Job drawing, mm, ordinate dimensions from the low corner. One solid piece. A direction names the side the tool comes from. Give positions to 0.01 mm unless a question says otherwise; leave off trailing zeros. Order: outer loops, then holes, each group sorted by start corner. A loop starts at its lowest first (then second) coordinate and runs counter-clockwise, first axis right, second up. Notation, with made-up numbers: M 27,-38 L 41,-38 A7 cw 41,-25 Z; hole C -4,43 d5. An arc over 180 degrees is marked long. Put each result on its own line as item: value. Start each with the question number.
1) Cut at D-D (z = 7.25). Write the cut outline in (x, y) (3 decimals), and give its area (3 significant figures).
2) Tool access for the marked faces 1 and 2: list every direction of +Z, -Z, +X, -X, +Y, -Y with a clear straight run to the whole face (end or side of a thin tool).
3) Two-plate mould, pull along Y, no slides. Class the marked faces 3, 4, 5 and 6: released by +Y, released by -Y, zero draft, split by the parting line, or undercut.
4) Pin check, flat tips, straight feed: pin 1 (3 mm diameter, centred on x = 4, z = 6.5, fed in from -Y); pin 2 (3 mm diameter, centred on x = 16.5, z = 5, fed in from -Y); pin 3 (2 mm diameter, centred on y = 6, z = 5.5, fed in from -X). Stop position of each tip, or through.
5) Cut at C-C (z = 4.25). Write the cut outline in (x, y).
6) Drill centre lines: line 1 (Z direction, x = 7.5, y = 11); line 2 (Z direction, x = 13.75, y = 3.5); line 3 (X direction, y = 8.25, z = 2.25). Where is each one in solid material? Low to high. Write a range as [from, to].
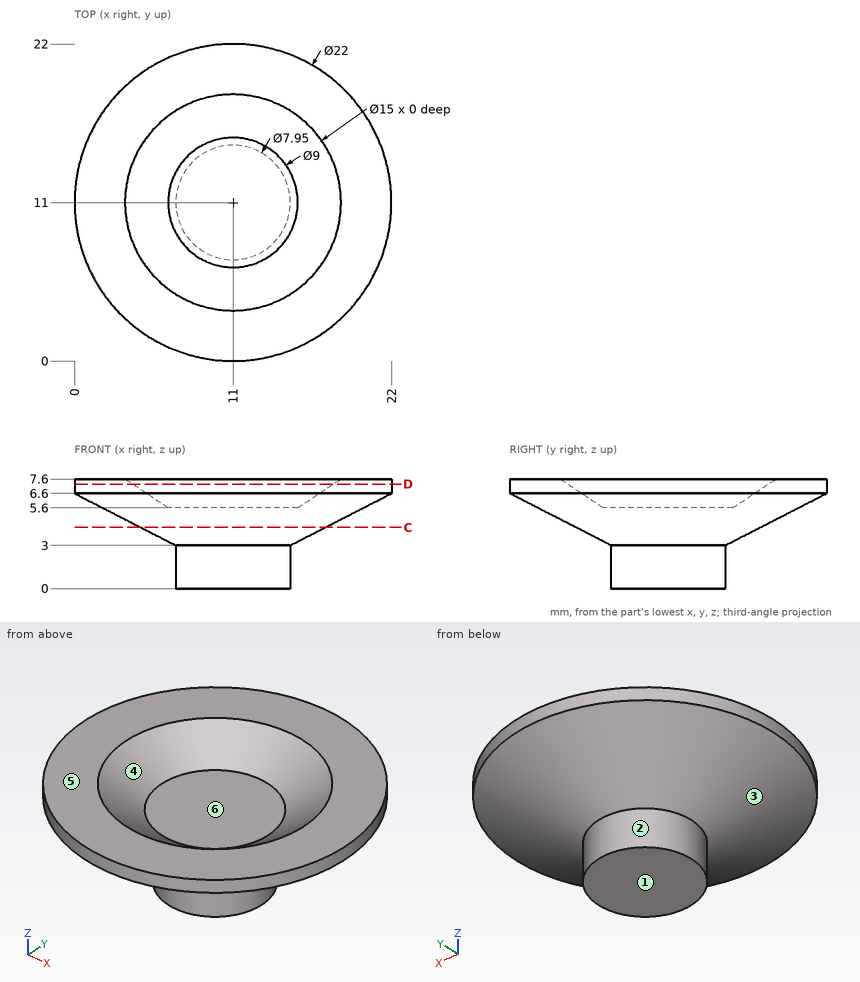
Solution:
1. outline: C 11,11 d22; hole C 11,11 d13.95
1. area: 227 mm²
2. face 1: -Z, +X, -X, +Y, -Y
2. face 2: -Z
3. face 3: split by the parting line
3. face 4: undercut
3. face 5: zero draft
3. face 6: undercut
4. pin 1: y = 1.48
4. pin 2: y = 1.59
4. pin 3: x = 1.36
5. outline: C 11,11 d12.83
6. line 1: [0, 5.6]
6. line 2: [5.06, 7.6]
6. line 3: [8.13, 13.87]
